```python
from build123d import *

# Parameters (mm, degrees)
BOSS_EXTRUDE1_DEPTH          = 18.5
SKETCH2_R                    = 6.3
CUT_EXTRUDE1_DEPTH           = 3.76
F_3_0_3_DIAMETER_HOLE1_D     = 3
F_3_0_3_DIAMETER_HOLE1_DEPTH = 10
F_3_0_3_DIAMETER_HOLE1_TIP   = 0.901290929
CUT_EXTRUDE2_DEPTH           = 3.76


with BuildPart() as part:
    # Sketch1 → Boss-Extrude1 (new body, symmetric)
    with BuildSketch(Plane(origin=(0, 0, 0), x_dir=(0, 0, -1), z_dir=(1, 0, 0))):
        Polygon((0, 0), (0, 27.76), (2.76, 27.76), (2.76, 2.76), (27.76, 2.76), (27.76, 0), align=None)
    extrude(amount=BOSS_EXTRUDE1_DEPTH, both=True)

    # Sketch2 → Cut-Extrude1 (cut, through all)
    with BuildSketch(Plane(origin=(0, 0, -2.76), x_dir=(-1, 0, 0), z_dir=(0, 0, -1))):
        with Locations((0, 14.26)):
            Circle(SKETCH2_R)
    extrude(amount=-CUT_EXTRUDE1_DEPTH, mode=Mode.SUBTRACT)

    # Ø3.0 (3) Diameter Hole1
    with Locations(Plane(origin=(0, 0, -2.76), x_dir=(-1, 0, 0), z_dir=(0, 0, -1))):
        with Locations((15.5, 21.26), (7.75, 7.836606241), (-7.75, 7.836606241), (-15.5, 21.26)):
            Hole(F_3_0_3_DIAMETER_HOLE1_D / 2, depth=F_3_0_3_DIAMETER_HOLE1_DEPTH)
            with Locations((0, 0, -(F_3_0_3_DIAMETER_HOLE1_DEPTH + F_3_0_3_DIAMETER_HOLE1_TIP / 2))):  # 118° drill point
                Cone(0, F_3_0_3_DIAMETER_HOLE1_D / 2, F_3_0_3_DIAMETER_HOLE1_TIP, mode=Mode.SUBTRACT)

    # Sketch5 → Cut-Extrude2 (cut, through all)
    with BuildSketch(Plane(origin=(0, 2.76, 0), x_dir=(1, 0, 0), z_dir=(0, 1, 0))):
        with BuildLine():
            Line((-13, 24.565), (-9, 24.565))
            ThreePointArc((-9, 24.565), (-7.445, 23.01), (-9, 21.455))
            Line((-9, 21.455), (-13, 21.455))
            ThreePointArc((-13, 21.455), (-14.555, 23.01), (-13, 24.565))
        make_face()
        with BuildLine():
            Line((-13, 11.065), (-9, 11.065))
            ThreePointArc((-9, 11.065), (-7.445, 9.51), (-9, 7.955))
            Line((-9, 7.955), (-13, 7.955))
            ThreePointArc((-13, 7.955), (-14.555, 9.51), (-13, 11.065))
        make_face()
        with BuildLine():
            Line((9, 11.065), (13, 11.065))
            ThreePointArc((13, 11.065), (14.555, 9.51), (13, 7.955))
            Line((13, 7.955), (9, 7.955))
            ThreePointArc((9, 7.955), (7.445, 9.51), (9, 11.065))
        make_face()
        with BuildLine():
            Line((9, 24.565), (13, 24.565))
            ThreePointArc((13, 24.565), (14.555, 23.01), (13, 21.455))
            Line((13, 21.455), (9, 21.455))
            ThreePointArc((9, 21.455), (7.445, 23.01), (9, 24.565))
        make_face()
    extrude(amount=-CUT_EXTRUDE2_DEPTH, mode=Mode.SUBTRACT)


solid = part.part
```
CAD build for the part. Positions are in the model's coordinates, mm. A direction names the side the tool comes from. Give positions to 0.01 mm unless a question says otherwise; leave off trailing zeros. Order: outer loops, then holes, each group sorted by start corner. A loop starts at its lowest first (then second) coordinate and runs counter-clockwise, first axis right, second up. Notation, with made-up numbers: M -19,11.5 L 29,11.5 A28 ccw 29,49.5 Z; hole C -21,-6.5 d1. An arc over 180 degrees is marked long. Put each result on its own line as item: value. Start each with the question number.
(1) Flat gauge pins, fed straight in: pin 1 Ø3 at (x, y) = (11.5, 15.5) entering from -Z; pin 2 Ø7.5 at (x, z) = (-5, -12.5) entering from +Y. Where does each tip first touch, or does it go through?
(2) Saw through at A-A, the plane x = -12.5. Write the cut outline in (y, z) (3 decimals).
(3) Saw through at D-D, the plane x = 0. Write the cut outline in (y, z), then the cut area to 3 significant figures.
(4) Drill centre lines: line 1 along Y through (x, z) = (7.75, -0.75); line 2 along Y through (x, z) = (-15.5, -1.4); line 3 along Z through (x, y) = (4, 26.75). Where is each one in solid material? Low to high.
(5) Saw through at B-B, the plane y = 21.26. Write the cut outline in (x, z).
(6) Which spindle directions (+Z, -Z, +X, -X, +Y, -Y) get a long thin tool onto all of the face, cutting with end or side? Do faces 3 (the flat face through (11, 1, -24.565)), 4 (the flat face through (0.3, 7.5, 0)). Say none if no direction does.
(7) Mould opens along Y. For faces 1 (the flat face through (0, 21, -2.76)), 2 (the cylindrical face through (6.644, 8.85, -1.361)) say: +Y half, -Y half, draft (parallel to the pull), parting line (faces both ways), or undercut.
(8) Saw through at C-C, the plane z = -9.51. Write the cut outline in (x, y) (3 decimals), then the cut area to 3 significant figures.
Check result:
1. pin 1: stops at z = -2.76
1. pin 2: stops at y = 2.76
2. outline: M 0,-27.76 L 2.76,-27.76 L 2.76,-24.565 L 0,-24.565 Z; M 0,-21.455 L 2.76,-21.455 L 2.76,-11.065 L 0,-11.065 Z; M 0,-7.955 L 2.76,-7.955 L 2.76,-2.76 L 27.76,-2.76 L 27.76,0 L 0,0 Z
3. outline: M 0,-27.76 L 2.76,-27.76 L 2.76,-2.76 L 7.96,-2.76 L 7.96,0 L 0,0 Z; M 20.56,-2.76 L 27.76,-2.76 L 27.76,0 L 20.56,0 Z
3. area: 111 mm2
4. line 1: y = 0 to 6.34, 9.34 to 27.76
4. line 2: y = 0 to 19.76, 22.76 to 27.76
4. line 3: z = -2.76 to 0
5. outline: M -18.5,-2.76 L -17,-2.76 L -17,0 L -18.5,0 Z; M -14,-2.76 L 14,-2.76 L 14,0 L -14,0 Z; M 17,-2.76 L 18.5,-2.76 L 18.5,0 L 17,0 Z
6. face 3: +Y, -Y
6. face 4: +Z, +X, -X, +Y, -Y
7. face 1: draft
7. face 2: undercut
8. outline: M -18.5,0 L -14.555,0 L -14.555,2.76 L -18.5,2.76 Z; M -7.445,0 L 7.445,0 L 7.445,2.76 L -7.445,2.76 Z; M 14.555,0 L 18.5,0 L 18.5,2.76 L 14.555,2.76 Z
8. area: 62.9 mm2
